```python
from build123d import *

# Parameters (mm, degrees)
SKETCH1_W                = 159.078855478
SKETCH1_H                = 159.078855478
BOSS_EXTRUDE1_DEPTH      = 38.1
BOSS_EXTRUDE1_DEPTH_BACK = 59.182
BOSS_EXTRUDE3_START      = 38.1
SKETCH1_5_R              = 11.43
BOSS_EXTRUDE3_DEPTH      = 5.08
SKETCH3_R                = 1.6
CUT_EXTRUDE1_DEPTH       = 163.124640459
FILLET4_R                = 5.08
SKETCH4_R                = 2.1
CUT_EXTRUDE2_DEPTH       = 5.08
SKETCH5_R                = 2.54
SKETCH5_R_2              = 4
SKETCH5_W                = 19
SKETCH5_H                = 12.5
CUT_EXTRUDE3_DEPTH       = 9.360572261
SKETCH7_W                = 25.4
SKETCH7_H                = 5.08
CUT_EXTRUDE4_DEPTH       = 5.588
BOSS_EXTRUDE4_DEPTH      = 25.4
CUT_EXTRUDE5_DEPTH       = 25.4
SKETCH11_W               = 12.7
SKETCH11_H               = 4.572
CUT_EXTRUDE6_DEPTH       = 5.334


with BuildPart() as part:
    # Sketch1 → Boss-Extrude1 (new, two sides)
    with BuildSketch(Plane(origin=(0, 0, 0), x_dir=(1, 0, 0), z_dir=(0, 1, 0))) as boss_extrude1_sk:
        with BuildLine():
            Line((-83.82, -88.9), (83.82, -88.9))
            ThreePointArc((83.82, -88.9), (87.412102448, -87.412102448), (88.9, -83.82))
            Line((88.9, -83.82), (88.9, 83.82))
            ThreePointArc((88.9, 83.82), (87.412102448, 87.412102448), (83.82, 88.9))
            Line((83.82, 88.9), (-83.82, 88.9))
            ThreePointArc((-83.82, 88.9), (-87.412102448, 87.412102448), (-88.9, 83.82))
            Line((-88.9, 83.82), (-88.9, -83.82))
            ThreePointArc((-88.9, -83.82), (-87.412102448, -87.412102448), (-83.82, -88.9))
        make_face()
        Rectangle(SKETCH1_W, SKETCH1_H, mode=Mode.SUBTRACT)
    extrude(amount=BOSS_EXTRUDE1_DEPTH)
    extrude(boss_extrude1_sk.sketch, amount=-BOSS_EXTRUDE1_DEPTH_BACK)

    # Sketch1<5> → Boss-Extrude3 (add)
    with BuildSketch(Plane(origin=(0, 0, 0), x_dir=(1, 0, 0), z_dir=(0, 1, 0)).offset(BOSS_EXTRUDE3_START)):
        with BuildLine():
            ThreePointArc((-88.9, -83.82), (-87.412102448, -87.412102448), (-83.82, -88.9))
            Line((-83.82, -88.9), (83.82, -88.9))
            ThreePointArc((83.82, -88.9), (87.412102448, -87.412102448), (88.9, -83.82))
            Line((88.9, -83.82), (88.9, 83.82))
            ThreePointArc((88.9, 83.82), (87.412102448, 87.412102448), (83.82, 88.9))
            Line((83.82, 88.9), (-83.82, 88.9))
            ThreePointArc((-83.82, 88.9), (-87.412102448, 87.412102448), (-88.9, 83.82))
            Line((-88.9, 83.82), (-88.9, -83.82))
        make_face()
        with Locations(Location((0, 0, 0), (0, 0, 270))):
            Circle(SKETCH1_5_R, mode=Mode.SUBTRACT)
    extrude(amount=BOSS_EXTRUDE3_DEPTH)

    # Sketch3 → Cut-Extrude1 (cut, through all)
    with BuildSketch(Plane(origin=(0, 43.18, 0), x_dir=(1, 0, 0), z_dir=(0, 1, 0))):
        with Locations(Location((-15.5, 15.5, 0), (0, 0, 270))):
            Circle(SKETCH3_R)
        with Locations(Location((-15.5, -15.5, 0), (0, 0, 270))):
            Circle(SKETCH3_R)
        with Locations(Location((15.5, 15.5, 0), (0, 0, 270))):
            Circle(SKETCH3_R)
        with Locations(Location((15.5, -15.5, 0), (0, 0, 270))):
            Circle(SKETCH3_R)
    extrude(amount=-CUT_EXTRUDE1_DEPTH, mode=Mode.SUBTRACT)

    # Fillet4
    fillet4_edges = [part.edges().sort_by_distance(p)[0] for p in [
        (79.539427739, -10.541, -79.539427739),
        (-79.539427739, -10.541, -79.539427739),
        (-79.539427739, -10.541, 79.539427739),
        (79.539427739, -10.541, 79.539427739),
    ]]
    fillet(fillet4_edges, radius=FILLET4_R)

    # Sketch4 → Cut-Extrude2 (cut)
    with BuildSketch(Plane(origin=(0, 43.18, 0), x_dir=(1, 0, 0), z_dir=(0, 1, 0))):
        with Locations(Location((-40.66, 40.66, 0), (0, 0, 270))):
            Circle(SKETCH4_R)
        with Locations(Location((40.66, 40.66, 0), (0, 0, 270))):
            Circle(SKETCH4_R)
        with Locations(Location((-40.66, -40.66, 0), (0, 0, 270))):
            Circle(SKETCH4_R)
        with Locations(Location((40.66, -40.66, 0), (0, 0, 270))):
            Circle(SKETCH4_R)
    extrude(amount=-CUT_EXTRUDE2_DEPTH, mode=Mode.SUBTRACT)

    # Sketch5 → Cut-Extrude3 (cut)
    with BuildSketch(Plane.XY.offset(88.9)):
        with Locations((-33.187618463, -11.513006866)):
            Circle(SKETCH5_R)
        with Locations((-33.187618463, 1.206455413)):
            Circle(SKETCH5_R)
        with Locations((-55.102312512, -31.62532479)):
            Circle(SKETCH5_R_2)
        with Locations((-55.584910431, -11.513006866)):
            Rectangle(SKETCH5_W, SKETCH5_H)
    extrude(amount=-CUT_EXTRUDE3_DEPTH, mode=Mode.SUBTRACT)

    # Sketch7 → Cut-Extrude4 (cut)
    with BuildSketch(Plane.XZ.offset(59.182)):
        with Locations((0, -82.079427739)):
            Rectangle(SKETCH7_W, SKETCH7_H)
    extrude(amount=-CUT_EXTRUDE4_DEPTH, mode=Mode.SUBTRACT)

    # Sketch10 → Boss-Extrude4 (add)
    with BuildSketch(Plane.ZY.offset(-12.7)):
        Polygon((-79.539427739, -46.736), (-79.539427739, -49.53), (-81.063427739, -49.53), align=None)
    extrude(amount=BOSS_EXTRUDE4_DEPTH)

    # Sketch10<2> → Cut-Extrude5 (cut)
    with BuildSketch(Plane.ZY.offset(-12.7)):
        Polygon((-79.539427739, -46.736), (-79.539427739, -49.53), (-81.063427739, -49.53), align=None)
    extrude(amount=CUT_EXTRUDE5_DEPTH, mode=Mode.SUBTRACT)

    # Sketch11 → Cut-Extrude6 (cut)
    with BuildSketch(Plane(origin=(0, 0, 79.539427739), x_dir=(-1, 0, 0), z_dir=(0, 0, -1))):
        with Locations((-44.45, -51.816)):
            Rectangle(SKETCH11_W, SKETCH11_H)
        with Locations((44.45, -51.816)):
            Rectangle(SKETCH11_W, SKETCH11_H)
    extrude(amount=-CUT_EXTRUDE6_DEPTH, mode=Mode.SUBTRACT)


solid = part.part
```
Design review of the part built by this model. Coordinates are the model's own, in mm. A direction names the side the tool comes from. Give positions to 0.01 mm unless a question says otherwise; leave off trailing zeros. Order: outer loops, then holes, each group sorted by start corner. A loop starts at its lowest first (then second) coordinate and runs counter-clockwise, first axis right, second up. Notation, with made-up numbers: (42, -38.75) -> (95, -38.75) arc R6 ccw to (95, -31.75) -> close; hole circle Ø5 at (-6.75, 72). An arc over 180 degrees is marked (long way). Write each question's results on one line, items separated by ' | '. Start each with the question number.
Q1. Mouldability with a two-part tool opening along Y and no side actions: class faces 6 (the flat face through (19, 43.18, -1)), 7 (the flat face through (88.9, -9, 1)), 8 (the flat face through (-65.085, -12, 84)) as +Y half, -Y half, draft (parallel to the pull), parting line (faces both ways), or undercut.
Q2. Add section B-B on x = 0. Give the boundary of the cut face in (y, z).
Q3. Add section D-D on x = 20.5. Give the boundary of the cut face in (y, z), and give its area (3 significant figures).
Q4. For pin 1 (4 mm diameter, centred on x = -63, z = 38, fed in from -Y); pin 2 (1.9 mm diameter, centred on x = 15.5, z = 15.5, fed in from -Y), all flat-tipped, find the tip position at first contact; note any pin that passes through.
Q5. Add section C-C on z = 1. Give the boundary of the cut face in (x, y), and give its area (3 significant figures).
Q6. Wall thickness on L1, parallel to X at y = 39.9, z = 15.5; L2, parallel to Z at x = -6.5, y = 27.5: over which ranges is each line inside the solid? List them lowest first. Write a range as from..to.
Q7. Add section A-A on y = 19. Give the boundary of the cut face in (x, z).
Q8. Machinability: for faces 1 (the flat face through (45, -49.53, 82)), 2 (the flat face through (-56, -5.263, 84)), 3 (the flat face through (-1, -9, 88.9)), 4 (the flat face through (12.7, -56, -82)), 5 (the cylindrical face through (87.451, -8.718, -87.372)), which of the approach directions +Z, -Z, +X, -X, +Y, -Y give a long, thin tool a straight path to every point of the face, cutting with its end or side? Answer none if there is none.
Found:
1) face 6: +Y half | face 7: draft | face 8: undercut
2) outline: (-59.18, -88.9) -> (43.18, -88.9) -> (43.18, -11.43) -> (38.1, -11.43) -> (38.1, -79.54) -> (-46.74, -79.54) -> (-49.53, -81.06) -> (-49.53, -79.54) -> (-53.59, -79.54) -> (-53.59, -84.62) -> (-59.18, -84.62) -> close; (-59.18, 79.54) -> (38.1, 79.54) -> (38.1, 11.43) -> (43.18, 11.43) -> (43.18, 88.9) -> (-59.18, 88.9) -> close
3) outline: (-59.18, -88.9) -> (43.18, -88.9) -> (43.18, 88.9) -> (-59.18, 88.9) -> (-59.18, 79.54) -> (38.1, 79.54) -> (38.1, -79.54) -> (-59.18, -79.54) -> close | area: 2,720 mm2
4) pin 1: stops at y = 38.1 | pin 2: passes through
5) outline: (-88.9, -59.18) -> (-79.54, -59.18) -> (-79.54, 38.1) -> (-11.39, 38.1) -> (-11.39, 43.18) -> (-88.9, 43.18) -> close; (11.39, 38.1) -> (79.54, 38.1) -> (79.54, -59.18) -> (88.9, -59.18) -> (88.9, 43.18) -> (11.39, 43.18) -> close | area: 2,610 mm2
6) L1: x = -88.9..-17.1, -13.9..13.9, 17.1..88.9 | L2: z = -88.9..-79.54, 79.54..88.9
7) outline: (-88.9, -83.82) arc R5.08 ccw to (-83.82, -88.9) -> (83.82, -88.9) arc R5.08 ccw to (88.9, -83.82) -> (88.9, 83.82) arc R5.08 ccw to (83.82, 88.9) -> (-83.82, 88.9) arc R5.08 ccw to (-88.9, 83.82) -> close; hole (-79.54, -74.46) arc R5.08 ccw to (-74.46, -79.54) -> (74.46, -79.54) arc R5.08 ccw to (79.54, -74.46) -> (79.54, 74.46) arc R5.08 ccw to (74.46, 79.54) -> (-74.46, 79.54) arc R5.08 ccw to (-79.54, 74.46) -> close
8) face 1: none | face 2: +Z | face 3: +Z, +X, -X, +Y, -Y | face 4: -Y | face 5: -Z, +X, +Y, -Y
